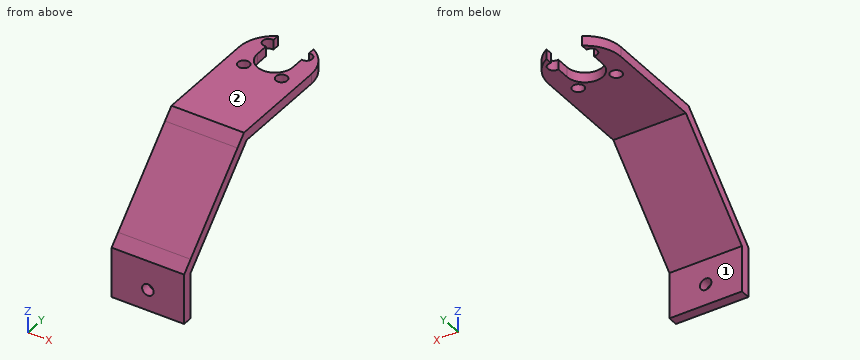
```python
from build123d import *

# Parameters (mm, degrees)
SKETCH1_R           = 1.75
BOSS_EXTRUDE1_DEPTH = 3
BOSS_EXTRUDE2_DEPTH = 3
SKETCH4_W           = 40
SKETCH4_H           = 3
BOSS_EXTRUDE3_DEPTH = 22
SKETCH5_R           = 1.75
CUT_EXTRUDE1_DEPTH  = 10
BOSS_EXTRUDE4_DEPTH = 1
BOSS_EXTRUDE5_DEPTH = 22
CUT_EXTRUDE2_DEPTH  = 75.598927606


# Read off the part's stored shape, not the designer's step: Boss-Extrude2
with BuildPart() as part:
    # Sketch1 → Boss-Extrude1 (new body)
    with BuildSketch(Plane.XY):
        with BuildLine():
            Line((5.4, 4.03535718), (5.4, 0))
            ThreePointArc((5.4, 0), (0, -5.4), (-5.4, 0))
            Line((-5.4, 0), (-5.4, 4.03535718))
            ThreePointArc((-5.4, 4.03535718), (-7.5, 5.75), (-5.4, 7.46464282))
            Line((-5.4, 7.46464282), (-5.4, 9.583318841))
            ThreePointArc((-5.4, 9.583318841), (0, -11), (5.4, 9.583318841))
            Line((5.4, 9.583318841), (5.4, 7.46464282))
            ThreePointArc((5.4, 7.46464282), (6.856797181, 7.105544171), (7.5, 5.75))
            ThreePointArc((7.5, 5.75), (6.856797181, 4.394455829), (5.4, 4.03535718))
        make_face()
        with Locations((-5.75, -5.75)):
            Circle(SKETCH1_R, mode=Mode.SUBTRACT)
        with Locations((5.75, -5.75)):
            Circle(SKETCH1_R, mode=Mode.SUBTRACT)
    extrude(amount=BOSS_EXTRUDE1_DEPTH)

    # Boss-Extrude2 outline → Boss-Extrude2 (add)
    with BuildSketch(Plane.XY):
        with BuildLine():
            Line((-11, 0), (-11, -59))
            Line((-11, -59), (11, -59))
            Line((11, -59), (11, 0))
            ThreePointArc((11, 0), (0, -11), (-11, 0))
        make_face()
    extrude(amount=BOSS_EXTRUDE2_DEPTH)

    # Sketch4 → Boss-Extrude3 (add)
    with BuildSketch(Plane.ZY.offset(11)):
        with Locations((-20, -57.5)):
            Rectangle(SKETCH4_W, SKETCH4_H)
    extrude(amount=-BOSS_EXTRUDE3_DEPTH)

    # Sketch5 → Cut-Extrude1 (cut)
    with BuildSketch(Plane(origin=(0, -59, 0), x_dir=(-1, 0, 0), z_dir=(0, -1, 0))):
        with Locations(Location((0, 33.63, 0), (0, 0, 90))):
            Circle(SKETCH5_R)
    extrude(amount=-CUT_EXTRUDE1_DEPTH, mode=Mode.SUBTRACT)

    # Sketch6 → Boss-Extrude4 (add)
    with BuildSketch(Plane.ZY.offset(11)):
        Polygon((-20, -56), (0, -36), (0, -56), align=None)
    boss_extrude4 = extrude(amount=-BOSS_EXTRUDE4_DEPTH)

    # Mirror1: Boss-Extrude4 across plane
    add(boss_extrude4.mirror(Plane(origin=(0, 0, 0), x_dir=(0, 0, 1), z_dir=(1, 0, 0))))

    # Sketch7 → Boss-Extrude5 (add, through all)
    with BuildSketch(Plane(origin=(11, 0, 0), x_dir=(0, 0, -1), z_dir=(1, 0, 0))):
        Polygon((0, -30), (26, -56), (21.757359313, -56), (0, -34.242640687), align=None)
    extrude(amount=-BOSS_EXTRUDE5_DEPTH)

    # Sketch8 → Cut-Extrude2 (cut, through all)
    with BuildSketch(Plane(origin=(11, 0, 0), x_dir=(0, 0, -1), z_dir=(1, 0, 0))):
        Polygon((10.878679656, -45.121320344), (24.757359313, -59), (-3, -59), (-3, -31.242640687), align=None)
    extrude(amount=-CUT_EXTRUDE2_DEPTH, mode=Mode.SUBTRACT)


solid = part.part
```
Geometry check sheet. Reference: the model listing, model coordinates, mm. Face numbers are marked on the shaded views. A direction names the side the tool comes from. Coordinates: 2 decimals unless noted, no trailing zeros. Write each loop counter-clockwise with the first axis right and the second up, starting at its lowest first coordinate (ties: lowest second). Pieces come first, ordered by that corner, then holes. Notation, with made-up numbers: M 32,30 L 81,30 A24 ccw 81,68 Z; hole C 54,-24 d6. An arc over 180 degrees is marked long. Use one line per item in the form item = value. Start each with the question number.
1) Section check B-B on x = 0. Enter the section's corners in (y, z), and give its area (3 significant figures).
2) Section check A-A on z = -33.63. Enter the section's corners in (x, y).
3) Section check D-D on y = -17.5. Enter the section's corners in (x, z).
4) Go/stop test with flat-tipped pins: pin 1 Ø1.5 at (y, z) = (2.5, 2) entering from -X; pin 2 Ø0.6 at (y, z) = (8.5, 1) entering from +X; pin 3 Ø4 at (x, z) = (8, -3) entering from +Y. Record where each tip stops, or that it passes through.
5) Set-up check for the marked faces 1 and 2: record each of +Z, -Z, +X, -X, +Y, -Y from which the full face is reachable in a straight line by a thin tool's end or side.
6) Thickness scan on probe 1 along Y at (x, z) = (-5.75, 1.5); probe 2 along Y at (x, z) = (-5.75, 1.6); probe 3 along X at (y, z) = (5.75, 1.1). Record the ranges inside material, lowest first. Write a range as from..to.
7) Section check C-C on x = -3. Enter the section's corners in (y, z).
Responses:
q1.outline = M -59,-40 L -56,-40 L -56,-35.38 L -59,-35.38 Z; M -59,-31.88 L -56,-31.88 L -56,-26 L -30,0 L -5.4,0 L -5.4,3 L -31.24,3 L -59,-24.76 Z
q1.area = 223 mm2
q2.outline = M -11,-59 L -1.75,-59 L -1.75,-56 L -11,-56 Z; M 1.75,-59 L 11,-59 L 11,-56 L 1.75,-56 Z
q3.outline = M -11,0 L 11,0 L 11,3 L -11,3 Z
q4.pin_1 = -10.86
q4.pin_2 = 7.33
q4.pin_3 = -31
q5.face_1 = -Z, +X, -X, +Y
q5.face_2 = +Z, +X, -X, +Y, -Y
q6.probe_1 = -32.74..-7.5, -4..4, 7.5..9.38
q6.probe_2 = -32.64..-7.5, -4..4, 7.5..9.38
q6.probe_3 = -9.38..-7.5, 7.5..9.38
q7.outline = M -59,-40 L -56,-40 L -56,-26 L -30,0 L -4.49,0 L -4.49,3 L -31.24,3 L -59,-24.76 Z
